```python
from build123d import *

# Parameters (mm, degrees)
F0_W     = 40
F0_H     = 40
F1_DEPTH = 1500
F2_SIZE2 = 19.290422
F2_SIZE  = 53


with BuildPart() as f1:
    # F0 (on Top) → F1 (new body)
    with BuildSketch(Plane.XY):
        Rectangle(F0_W, F0_H)
    extrude(amount=-F1_DEPTH)

    # F2
    f2_edges = [f1.edges().sort_by_distance(p)[0] for p in [
        (0, -20, -1500),
        (20, 0, -1500),
        (0, 20, -1500),
        (-20, 0, -1500),
    ]]
    chamfer(f2_edges, length=F2_SIZE, length2=F2_SIZE2)


solid = f1.part
```
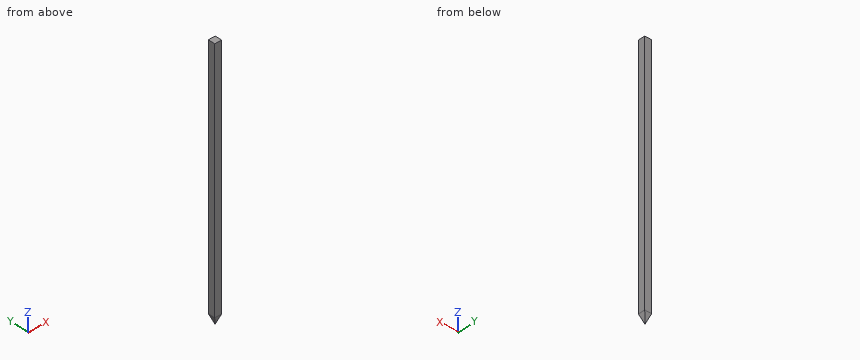
For this review, take the finished solid that the model builds, in its own axes (mm). Give positions to 0.01 mm unless a question says otherwise; leave off trailing zeros. Order: outer loops, then holes, each group sorted by start corner. A loop starts at its lowest first (then second) coordinate and runs counter-clockwise, first axis right, second up.
1) Take a section at A-A (x = 9). Give the boundary of the cut face in (y, z), then the cut area to 3 significant figures.
2) Insertion check: pin 1 (12 mm diameter, centred on x = 7, y = -11.5, fed in from -Z). The pin has a flat end and moves straight along its axis. Give the tip position at first contact, or say it passes through.
3) Take a section at B-B (y = -8.5). Give the boundary of the cut face in (x, z), then the cut area to 3 significant figures.
Derived:
1. outline: (-20, -1447) - (-9, -1477.22) - (9, -1477.22) - (20, -1447) - (20, 0) - (-20, 0) - close
1. area: 58,800 mm2
2. pin 1: stops at z = -1486.42
3. outline: (-20, -1447) - (-8.5, -1478.6) - (8.5, -1478.6) - (20, -1447) - (20, 0) - (-20, 0) - close
3. area: 58,800 mm2
